Drawing for the job (mm, zero at the part's lowest x, y, z). A direction names the side the tool comes from. Round coordinates to 2 decimals unless told otherwise and drop trailing zeros. Write each loop counter-clockwise with the first axis right and the second up, starting at its lowest first coordinate (ties: lowest second). Pieces come first, ordered by that corner, then holes. Notation, with made-up numbers: (43, -6.75) - (53, -6.75) arc R27 ccw to (53, 19.25) - close; hole circle Ø11 at (83, 15). An arc over 180 degrees is marked (long way). One line per question, with ' | ' between items.
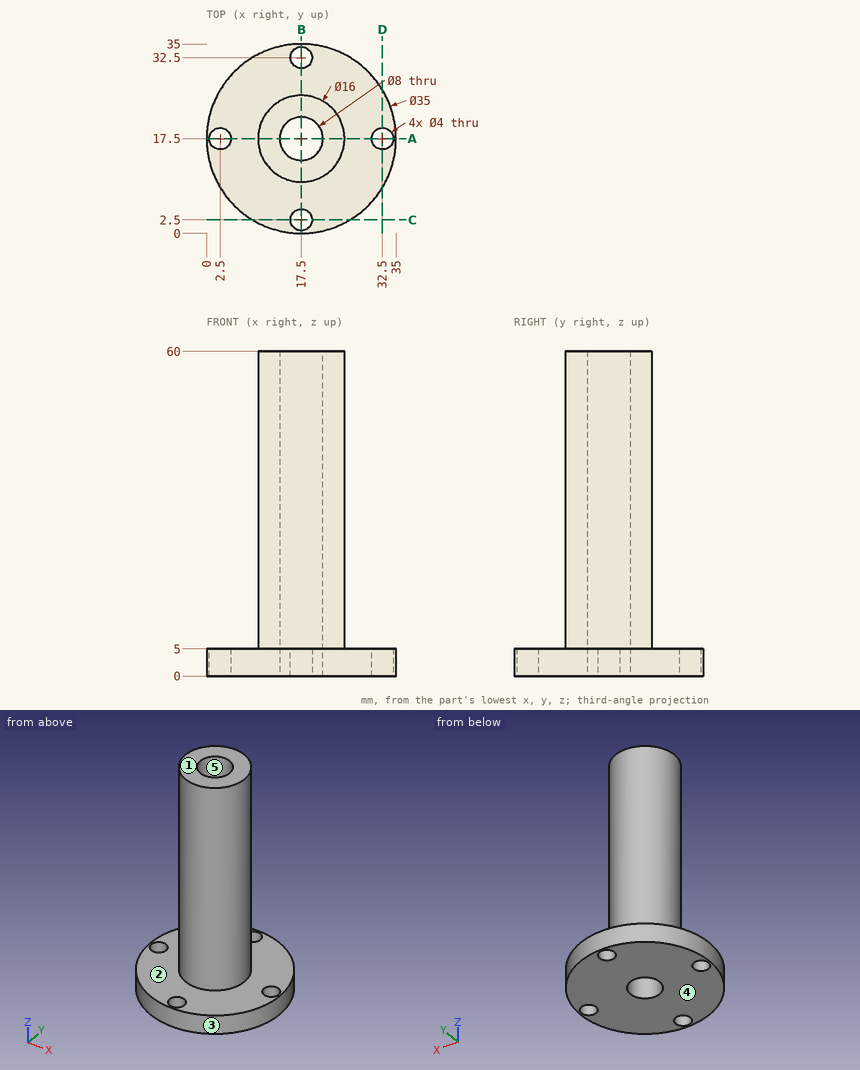
Q1. Which spindle directions (+Z, -Z, +X, -X, +Y, -Y) get a long thin tool onto all of the face, cutting with end or side? Do the marked faces 1 and 2. Say none if no direction does.
Found:
face 1: +Z, +X, -X, +Y, -Y | face 2: +Z
Q2. Drill centre lines: L1, parallel to Y at x = 17.5, z = 35; L2, parallel to Y at x = 17, z = 1; L3, parallel to Z at x = 31, y = 23. Where is each one in solid material? Low to high. Write a range as from..to.
Found:
L1: 9.5..13.5, 21.5..25.5 | L2: 0.01..0.56, 4.44..13.53, 21.47..30.56, 34.44..34.99 | L3: 0..5
Q3. Pull direction Y, two halves, no side cores. Call the marked faces 3, 4 and 5: +Y half, -Y half, draft (parallel to the pull), parting line (faces both ways), or undercut.
Found:
face 3: parting line | face 4: draft | face 5: undercut
Q4. Saw through at C-C, the plane y = 2.5. List the corners of the cut face in (x, z), then the cut area to 3 significant figures.
Found:
outline: (8.49, 0) - (15.5, 0) - (15.5, 5) - (8.49, 5) - close; (19.5, 0) - (26.51, 0) - (26.51, 5) - (19.5, 5) - close | area: 70.1 mm^2
Q5. Saw through at A-A, the plane y = 17.5. List the corners of the cut face in (x, z).
Found:
outline: (0, 0) - (0.5, 0) - (0.5, 5) - (0, 5) - close; (4.5, 0) - (13.5, 0) - (13.5, 60) - (9.5, 60) - (9.5, 5) - (4.5, 5) - close; (21.5, 0) - (30.5, 0) - (30.5, 5) - (25.5, 5) - (25.5, 60) - (21.5, 60) - close; (34.5, 0) - (35, 0) - (35, 5) - (34.5, 5) - close
Q6. Drop flat-ended pins along their axis: pin 1 (1.5 mm diameter, centred on x = 20, z = 44, fed in from -Y); pin 2 (2 mm diameter, centred on y = 11.5, z = 22.5, fed in from +X) (3 decimals); pin 3 (1 mm diameter, centred on x = 25, z = 9.5, fed in from -Y). Give the stop position or say it passes through.
Found:
pin 1: y = 9.69 | pin 2: x = 23.745 | pin 3: y = 13.63
